Drawing for the job (mm, zero at the part's lowest x, y, z). A direction names the side the tool comes from. Round coordinates to 2 decimals unless told otherwise and drop trailing zeros. Write each loop counter-clockwise with the first axis right and the second up, starting at its lowest first coordinate (ties: lowest second). Pieces come first, ordered by that corner, then holes.
Item 1: Band-saw the part on B-B, the plane z = 296.5. Write the cut outline in (x, y), then the cut area to 3 significant figures.
Item 2: Mould opens along Z. For the marked faces 3, 4 and 5 say: +Z half, -Z half, draft (parallel to the pull), parting line (faces both ways), or undercut.
Item 3: Band-saw the part on C-C, the plane y = 134. Write the cut outline in (x, z).
Item 4: 3-axis set-ups, long thin cutter, end or side, ignore diameter. For the marked faces 1 and 2: which of +Z, -Z, +X, -X, +Y, -Y reach the whole face in a straight line?
Item 5: Band-saw the part on A-A, the plane x = 430. Write the cut outline in (y, z), then the cut area to 3 significant figures.
Item 6: Wall check: probe 1 along Z at (x, y) = (447, 210.5); probe 2 along X at (y, z) = (80, 173); probe 3 along X at (y, z) = (250, 366). Give the ranges that are in metal, low to high.
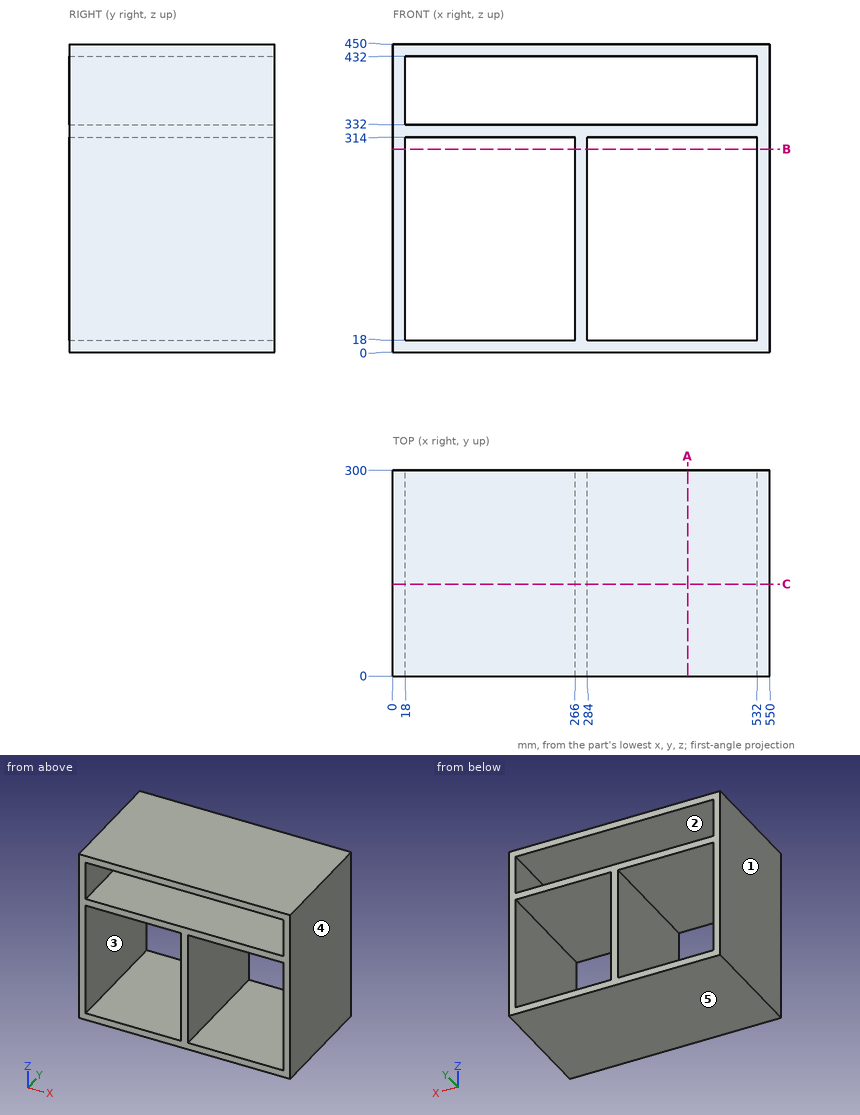
Results:
1. outline: (0, 0) - (18, 0) - (18, 300) - (0, 300) - close; (266, 0) - (284, 0) - (284, 300) - (266, 300) - close; (532, 0) - (550, 0) - (550, 300) - (532, 300) - close
1. area: 16,200 mm2
2. face 3: undercut
2. face 4: draft
2. face 5: -Z half
3. outline: (0, 0) - (550, 0) - (550, 450) - (0, 450) - close; hole (18, 18) - (266, 18) - (266, 314) - (18, 314) - close; hole (18, 332) - (532, 332) - (532, 432) - (18, 432) - close; hole (284, 18) - (532, 18) - (532, 314) - (284, 314) - close
4. face 1: +Z, -Z, -X, +Y, -Y
4. face 2: +Y, -Y
5. outline: (0, 0) - (300, 0) - (300, 18) - (0, 18) - close; (0, 314) - (300, 314) - (300, 332) - (0, 332) - close; (0, 432) - (300, 432) - (300, 450) - (0, 450) - close
5. area: 16,200 mm2
6. probe 1: z = 0 to 18, 314 to 332, 432 to 450
6. probe 2: x = 0 to 18, 266 to 284, 532 to 550
6. probe 3: x = 0 to 18, 532 to 550
